Can you work these out from the drawing? Everything is in mm from the part's minimum corner. A direction names the side the tool comes from. Coordinates: 2 decimals unless noted, no trailing zeros. Order: outer loops, then holes, each group sorted by start corner. A loop starts at its lowest first (then second) coordinate and runs counter-clockwise, first axis right, second up. Notation, with made-up numbers: (-10, 1.25) -> (1, 1.25) arc R4 cw to (1, 5.25) -> close; hole circle Ø8 at (84, 21.5). An arc over 180 degrees is marked (long way). Return JSON: item names as keys, results as strings. Group by question number.
1) If I drill on probe 1 along X at (y, z) = (7.75, 3); probe 2 along Z at (x, y) = (8, 3.75) (1 decimal); probe 3 along Z at (x, y) = (6, 3.25), over which ranges is the centre line in solid material (lowest first)? Write a range as from..to.
2) If we section it at A-A, the plane x = 8.75: Please give me the cut outline in (y, z), then the cut area to 3 significant figures.
3) For pin 1 (4 mm diameter, centred on x = 7.5, y = 4, fed in from +Z); pin 2 (4 mm diameter, centred on x = 6.5, y = 8, fed in from -Z) (1 decimal); pin 3 (4 mm diameter, centred on x = 7, z = 5, fed in from +Y), each with a flat end and sliding along its axis, tell me the tip position at first contact or that it passes through.
4) For the marked faces 1 and 2, which set-ups out of +Z, -Z, +X, -X, +Y, -Y let a thin tool reach every point of the face, with its end or its side?
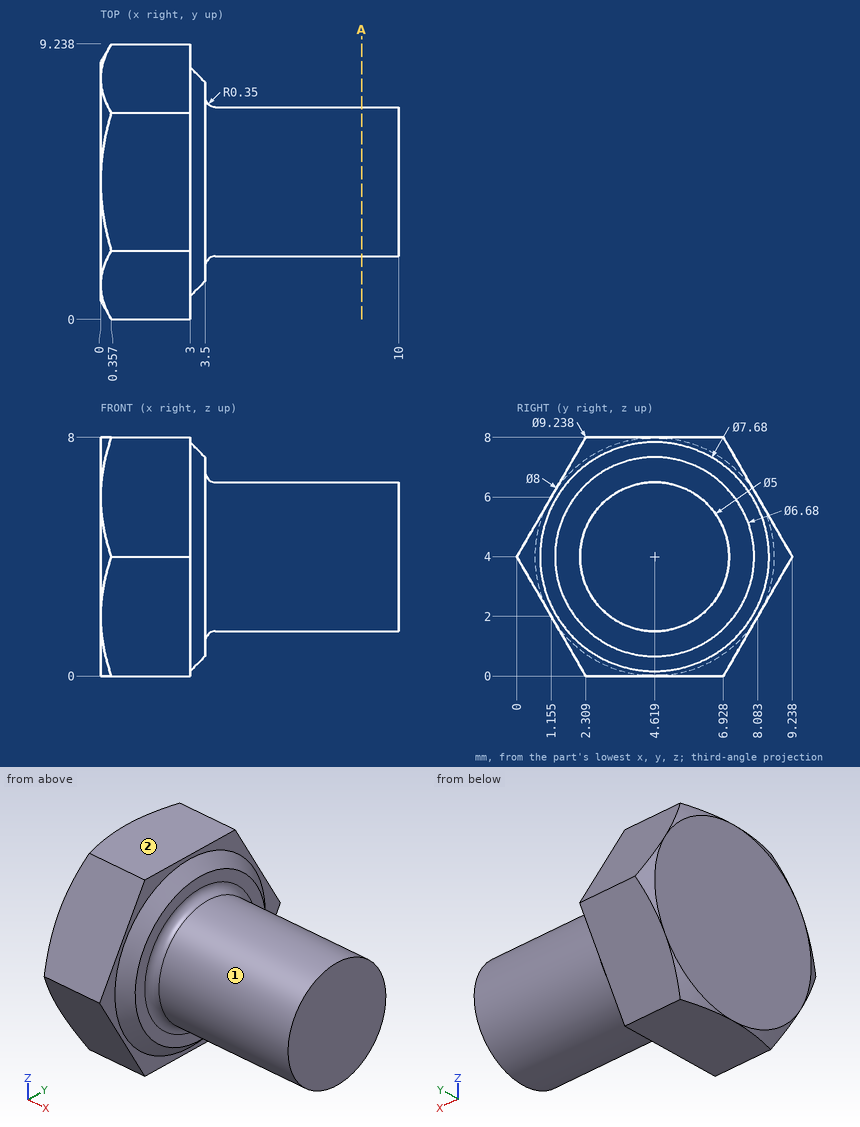
Result sheet:
{
 "1": {"probe 1": "x = 0..3.5", "probe 2": "z = 1.7..6.3", "probe 3": "z = 1.91..6.09"},
 "2": {"outline": "circle Ø5 at (4.62, 4)", "area": "19.6 mm2"},
 "3": {"pin 1": "stops at z = 6.5", "pin 2": "stops at z = 1.9", "pin 3": "stops at y = 7.12"},
 "4": {"face 1": "+X", "face 2": "+Z, +X, -X, +Y, -Y"}
}
